```python
from build123d import *

# Parameters (mm, degrees)
BOSS_EXTRU_1_DEPTH      = 100
ESQUISSE2_R             = 9
ESQUISSE2_W             = 50
ESQUISSE2_H             = 15
ENL_V_MAT_EXTRU_1_DEPTH = 100


with BuildPart() as part:
    # Esquisse1 → Boss.-Extru.1 (new body)
    with BuildSketch(Plane.XY):
        with BuildLine():
            Line((1005.392443992, 375.619056085), (1000.392443992, 375.619056085))
            Line((1000.392443992, 375.619056085), (1000.392443992, 322.619056085))
            Line((1000.392443992, 322.619056085), (1040.392443992, 322.619056085))
            Line((1040.392443992, 322.619056085), (1040.392443992, 375.619056085))
            Line((1040.392443992, 375.619056085), (1035.392443992, 375.619056085))
            ThreePointArc((1035.392443992, 375.619056085), (1020.392443992, 364.024180923), (1005.392443992, 375.619056085))
        make_face()
    extrude(amount=BOSS_EXTRU_1_DEPTH)

    # Esquisse2 → Enlèv. mat.-Extru.1 (cut)
    with BuildSketch(Plane(origin=(1040.392443992, 0, 0), x_dir=(0, 0, -1), z_dir=(1, 0, 0))):
        with Locations((-50, 337.619056085)):
            Circle(ESQUISSE2_R)
        with Locations((-50, 368.119056085)):
            Rectangle(ESQUISSE2_W, ESQUISSE2_H)
    extrude(amount=-ENL_V_MAT_EXTRU_1_DEPTH, mode=Mode.SUBTRACT)


solid = part.part
```
Could you check a few things on this model? Use its own coordinates, in mm. A direction names the side the tool comes from. Coordinates: 2 decimals unless noted, no trailing zeros. Order: outer loops, then holes, each group sorted by start corner. A loop starts at its lowest first (then second) coordinate and runs counter-clockwise, first axis right, second up. Notation, with made-up numbers: M 47.25,44.25 L 65.25,44.25 A23 cw 65.25,56.25 Z; hole C -18,32.5 d9. An arc over 180 degrees is marked long. Use one line per item in the form item = value. Start each with the question number.
1. Suppose I cut it at A-A on z = 50. Write out the boundary of the cut face in (x, y).
2. Suppose I cut it at D-D on z = 87. Write out the boundary of the cut face in (x, y).
3. Suppose I cut it at B-B on y = 332.5. Write out the boundary of the cut face in (x, z), then the cut area to 3 significant figures.
4. We'd pull the mould along Y, two halves only. Please class faces 3 (the cylindrical face through (1020.672, 343.702, 56.633)), 4 (the cylindrical face through (1020.678, 364.027, 12.325)), 5 (the flat face through (1000.392, 349, 49)), 6 (the flat face through (1020, 322.619, 49)): +Y half, -Y half, draft (parallel to the pull), parting line (faces both ways), or undercut.
5. On a 3-axis mill with a long thin cutter (end or side, diameter ignored), from which of +Z, -Z, +X, -X, +Y, -Y can I reach the whole of each face in a straight line? I mean faces 1 (the flat face through (1021, 360.619, 50)), 2 (the flat face through (1040.392, 349, 49)). Say none if no direction works.
6. Please list where these lines run through material, in increasing order: line 1 (Y direction, x = 1031, z = 50); line 2 (Z direction, x = 1006, y = 364); line 3 (Z direction, x = 1035, y = 345.5).
7. For pin 1 (5 mm diameter, centred on x = 1020.5, z = 57.5, fed in from +Y); pin 2 (12 mm diameter, centred on x = 1013, y = 369, fed in from -Z), each with a flat end and sliding along its axis, tell me the tip position at first contact or that it passes through.
8. Suppose I cut it at C-C on x = 1032. Write out the boundary of the cut face in (y, z), then the cut area to 3 significant figures.
Geometry says:
q1.outline = M 1000.39,322.62 L 1040.39,322.62 L 1040.39,328.62 L 1000.39,328.62 Z; M 1000.39,346.62 L 1040.39,346.62 L 1040.39,360.62 L 1000.39,360.62 Z
q2.outline = M 1000.39,322.62 L 1040.39,322.62 L 1040.39,375.62 L 1035.39,375.62 A15.5 cw 1005.39,375.62 L 1000.39,375.62 Z
q3.outline = M 1000.39,0 L 1040.39,0 L 1040.39,42.6 L 1000.39,42.6 Z; M 1000.39,57.4 L 1040.39,57.4 L 1040.39,100 L 1000.39,100 Z
q3.area = 3,410 mm^2
q4.face_3 = undercut
q4.face_4 = +Y half
q4.face_5 = draft
q4.face_6 = -Y half
q5.face_1 = +X, -X, +Y
q5.face_2 = +Z, -Z, +X, +Y, -Y
q6.line_1 = 322.62 to 328.62, 346.62 to 360.62
q6.line_2 = 0 to 25, 75 to 100
q6.line_3 = 0 to 45.65, 54.35 to 100
q7.pin_1 = 360.62
q7.pin_2 = 0
q8.outline = M 322.62,0 L 369.25,0 L 369.25,25 L 360.62,25 L 360.62,75 L 369.25,75 L 369.25,100 L 322.62,100 Z; hole C 337.62,50 d18
q8.area = 3,980 mm^2
